Work out the finished part from the listing and answer in its coordinate system (mm). A direction names the side the tool comes from. Give positions to 0.01 mm unless a question says otherwise; leave off trailing zeros. Write each loop counter-clockwise with the first axis right and the second up, starting at its lowest first coordinate (ties: lowest second). Pieces come first, ordered by that corner, then holes. Notation, with made-up numbers: (24, 32) - (58, 32) arc R8 ccw to (58, 46) - close; hole circle Ø11 at (-32.75, -29). An arc over 180 degrees is marked (long way). Write item = value, one per line.
from build123d import *

# Parameters (mm, degrees)
F1_DEPTH      = 150
F2_W          = 64.235858
F2_H          = 19.400093
F3_DEPTH      = 17
F3_DEPTH_BACK = 16


with BuildPart() as f1:
    # F0 (on Front) → F1 (new body)
    with BuildSketch(Plane.XZ):
        Polygon((-11.211432, 5.705079), (-16.532733, -6.356537), (15.868079, -7.066044), (10.428526, 7.242345), (5.698481, -3.44145), (-0.016305, 7.358057), (-4.234615, -3.44145), align=None)
    extrude(amount=F1_DEPTH)

    # F2 (on Top) → F3 (join, two sides)
    with BuildSketch(Plane.XY) as f3_sk:
        with Locations((-0.431113, -1.717609)):
            Rectangle(F2_W, F2_H)
    extrude(amount=F3_DEPTH)
    extrude(f3_sk.sketch, amount=-F3_DEPTH_BACK)


solid = f1.part
1. Find section C-C, the plane z = -12.5. Give the vertices of the cut face in (x, y), then the cut area to 3 significant figures.
Solution:
outline = (-32.55, -11.42) - (31.69, -11.42) - (31.69, 7.98) - (-32.55, 7.98) - close
area = 1,250 mm^2
2. Given pin 1 (1.5 mm diameter, centred on y = -46, z = -6, fed in from -X); pin 2 (16.5 mm diameter, centred on x = -2, z = 8, fed in from -Y); pin 3 (2 mm diameter, centred on x = 8.5, y = -49.5, fed in from -Z); pin 4 (2 mm diameter, centred on y = -79.5, z = 1.5, fed in from +X), each flat-ended and moving along its own axis, determine where each tip first touches the part or whether it passes through.
Solution:
pin_1 = -16.53
pin_2 = -150
pin_3 = -6.93
pin_4 = 12.99
3. Find section B-B, the plane x = 20.5. Give the vertices of the cut face in (y, z), then the cut area to 3 significant figures.
Solution:
outline = (-11.42, -16) - (7.98, -16) - (7.98, 17) - (-11.42, 17) - close
area = 640 mm^2
4. A tool of negligible diameter and unlimited length cuts with its end or side. For faces 1 (the flat face through (-13.835, -79.739, -0.241)), 2 (the flat face through (-1, -2, -16)), 3 (the flat face through (-2.096, -79.739, 2.034)), from which of +Z, -Z, +X, -X, +Y, -Y can it reach the whole face along a straight path? Write none if from no direction.
Solution:
face_1 = +Z, -X, -Y
face_2 = -Z, +X, -X, +Y, -Y
face_3 = +Z, -Y
5. Find section A-A, the plane y = -39.5. Give the vertices of the cut face in (x, z), then the cut area to 3 significant figures.
Solution:
outline = (-16.53, -6.36) - (15.87, -7.07) - (10.43, 7.24) - (5.7, -3.44) - (-0.02, 7.36) - (-4.23, -3.44) - (-11.21, 5.71) - close
area = 253 mm^2
6. Straight lines are drawn through the part: line 1 (X direction, y = -98, z = -0.5); line 2 (X direction, y = -52, z = 1); line 3 (Y direction, x = 12.5, z = 5.5). For each, find the intervals that lie inside material, in ascending order.
Solution:
line_1 = -13.95 to -6.48, -3.09 to 4.14, 7 to 13.37
line_2 = -13.29 to -7.62, -2.5 to 3.35, 7.66 to 12.8
line_3 = -11.42 to 7.98
7. For a pull along X with two mould halves and no side action, classify faces 4 (the flat face through (-32.549, -2, 1)), 5 (the flat face through (8.1, -79.74, 1.98)), 6 (the flat face through (13.186, -79.739, -0.012)), 7 (the flat face through (-1, 7.982, 1)) as pulls with the +X half, pulls with the -X half, needs draft (parallel to the pull), parting line crosses it, or undercut.
Solution:
face_4 = pulls with the -X half
face_5 = undercut
face_6 = pulls with the +X half
face_7 = needs draft
8. Find section D-D, the plane x = -2. Give the vertices of the cut face in (y, z), then the cut area to 3 significant figures.
Solution:
outline = (-150, -6.67) - (-11.42, -6.67) - (-11.42, -16) - (7.98, -16) - (7.98, 17) - (-11.42, 17) - (-11.42, 2.28) - (-150, 2.28) - close
area = 1,880 mm^2
